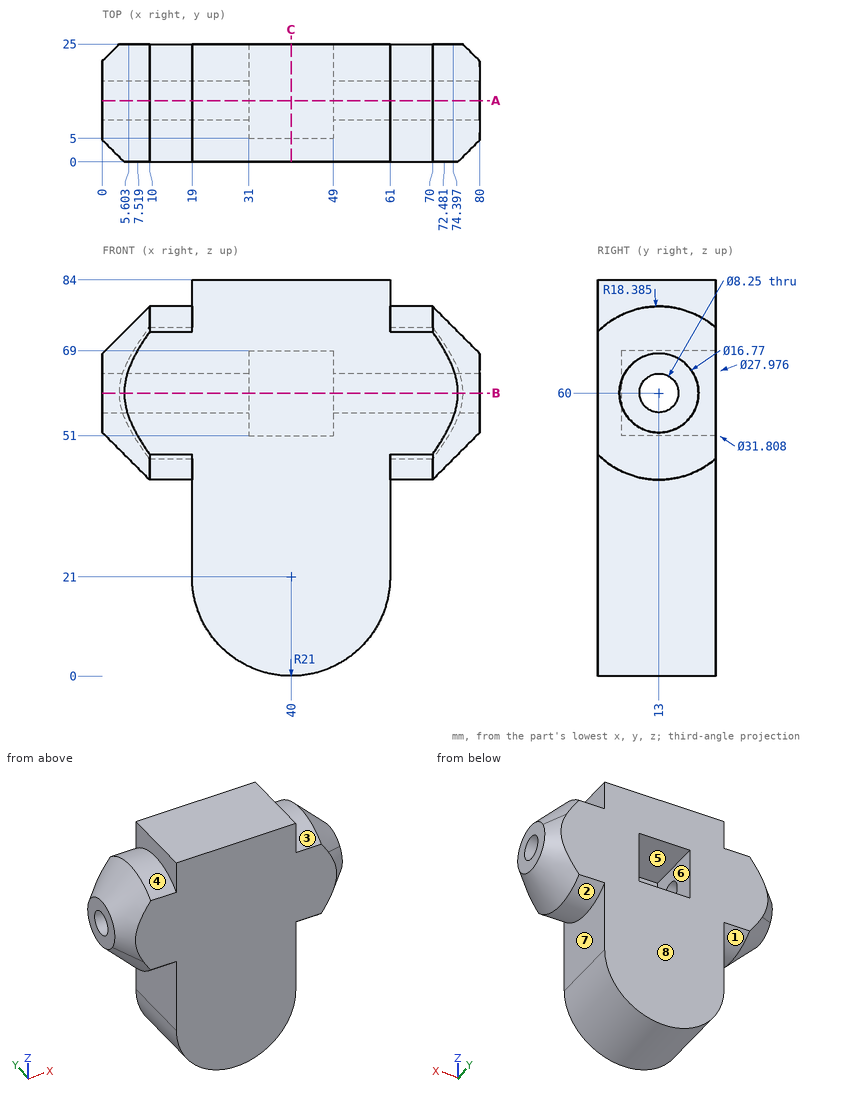
The drawing under review shows one solid part. Ordinate dimensions are in mm from its lowest x, y, z. A direction names the side the tool comes from. Coordinates: 2 decimals unless noted, no trailing zeros. Loops run counter-clockwise (first coordinate to the right, second up) from the corner with the lowest first, then second, coordinate; pieces in that order, holes last. Notation, with made-up numbers: (41.25, -32) - (45.25, -32) arc R19 ccw to (45.25, 4) - close; hole circle Ø4 at (3, 60.5). An arc over 180 degrees is marked (long way). Return JSON: item names as keys, results as strings.
Item 1: For line 1 (Y direction, x = 21, z = 60) (1 decimal); line 2 (X direction, y = 20.25, z = 62); line 3 (X direction, y = 16.5, z = 35.5), list the stretches that pass through material, from the lowest coordinate up.
Determined:
{"line 1": "y = 0 to 8.9, 17.1 to 25", "line 2": "x = 0 to 31, 49 to 80", "line 3": "x = 19 to 61"}
Item 2: Insertion check: pin 1 (9 mm diameter, centred on x = 43, z = 63.5, fed in from +Y); pin 2 (12 mm diameter, centred on y = 17.5, z = 77, fed in from -X); pin 3 (2 mm diameter, centred on y = 16, z = 37.5, fed in from -X). Each pin has a flat end and moves straight along its axis. Give the tip position at first contact, or say it passes through.
Determined:
{"pin 1": "stops at y = 5", "pin 2": "stops at x = 3.2", "pin 3": "stops at x = 19"}
Item 3: Take a section at C-C (x = 40). Give the boundary of the cut face in (y, z).
Determined:
{"outline": "(0, 0) - (25, 0) - (25, 51) - (5, 51) - (5, 69) - (25, 69) - (25, 84) - (0, 84) - close"}
Item 4: Take a section at A-A (y = 13). Give the boundary of the cut face in (x, z) (1 decimal), then the cut area to 3 significant figures.
Determined:
{"outline": "(0, 51.6) - (10, 41.6) - (19, 41.6) - (19, 21) arc R21 ccw to (61, 21) - (61, 41.6) - (70, 41.6) - (80, 51.6) - (80, 55.9) - (49, 55.9) - (49, 51) - (31, 51) - (31, 55.9) - (0, 55.9) - close; (0, 64.1) - (31, 64.1) - (31, 69) - (49, 69) - (49, 64.1) - (80, 64.1) - (80, 68.4) - (70, 78.4) - (61, 78.4) - (61, 84) - (19, 84) - (19, 78.4) - (10, 78.4) - (0, 68.4) - close", "area": "3,700 mm2"}
Item 5: For the marked faces 1, 2, 3, 4 and 5, list the 3-axis set-ups (+Z, -Z, +X, -X, +Y, -Y) from which the entire face can be reached by the end or side of a thin tool; tool diameter is ignored.
Determined:
{"face 1": "-Z, -X", "face 2": "-Z, +X", "face 3": "+Z, +X", "face 4": "+Z, -X", "face 5": "+Y"}
Item 6: Mouldability with a two-part tool opening along X and no side actions: class the marked faces 6, 7 and 8 as pulls with the +X half, pulls with the -X half, needs draft (parallel to the pull), parting line crosses it, or undercut.
Determined:
{"face 6": "undercut", "face 7": "pulls with the +X half", "face 8": "needs draft"}
Item 7: Take a section at B-B (z = 60). Give the boundary of the cut face in (x, y) (1 decimal), then the cut area to 3 significant figures.
Determined:
{"outline": "(0, 4.6) - (4.6, 0) - (75.4, 0) - (80, 4.6) - (80, 8.9) - (49, 8.9) - (49, 5) - (31, 5) - (31, 8.9) - (0, 8.9) - close; (0, 17.1) - (31, 17.1) - (31, 25) - (3.6, 25) - (0, 21.4) - close; (49, 17.1) - (80, 17.1) - (80, 21.4) - (76.4, 25) - (49, 25) - close", "area": "1,090 mm2"}
